Geometry check sheet. Reference: the model listing, model coordinates, mm. Round coordinates to 2 decimals unless told otherwise and drop trailing zeros. Order: outer loops, then holes, each group sorted by start corner. A loop starts at its lowest first (then second) coordinate and runs counter-clockwise, first axis right, second up. Notation, with made-up numbers: (-4, -19) - (43, -19) arc R10 cw to (43, -11) - close; hole circle Ø3 at (60.5, -18.5). An arc over 180 degrees is marked (long way). Return JSON: item names as keys, results as strings. Group by question number.
Q1. Draft check along X on faces 1 (the flat face through (5, 42, 88)), 2 (the cylindrical face through (-0.221, 63.686, 88.479)), 3 (the flat face through (0, 42, 90)). Enter one of: pulls with the +X half, pulls with the -X half, needs draft (parallel to the pull), parting line crosses it, or undercut.
Q2. Gauge pin test, flat end, axial feed: pin 1 Ø5.5 at (x, y) = (0, 22) entering from -Z. Record the tip position at first contact, or that the pin passes through.
Q3. Material ranges on line 1 along Y through (x, z) = (0, 89.2); line 2 along X through (y, z) = (22, 88.7); line 3 along Y through (x, z) = (1, 87.25), recorded low to high.
Q4. Sectioned sample at C-C, the plane z = 89.25. Record the cut outline in (x, y), then the cut area to 3 significant figures.
Q5. Sectioned sample at B-B, the plane x = 0. Record the cut outline in (y, z).
Q6. Sectioned sample at A-A, the plane y = 62. Record the cut outline in (x, z), then the cut area to 3 significant figures.
```python
from build123d import *

# Parameters (mm, degrees)
SKETCH1_W      = 10
SKETCH1_H      = 44
BAR_DEPTH      = 3
SKETCH2_R      = 1.7
M3_HOLES_DEPTH = 5


with BuildPart() as part:
    # Sketch1 → Bar (new body)
    with BuildSketch(Plane.XY.offset(87)):
        with Locations((0, 42)):
            Rectangle(SKETCH1_W, SKETCH1_H)
    extrude(amount=BAR_DEPTH)

    # Sketch2 → M3_holes (cut)
    with BuildSketch(Plane.XY.offset(86)):
        with Locations((0, 62)):
            Circle(SKETCH2_R)
        with Locations((0, 22)):
            Circle(SKETCH2_R)
    extrude(amount=M3_HOLES_DEPTH, mode=Mode.SUBTRACT)


solid = part.part
```
Reply:
{
 "1": {"face 1": "pulls with the +X half", "face 2": "undercut", "face 3": "needs draft"},
 "2": {"pin 1": "z = 87"},
 "3": {"line 1": "20 to 20.3, 23.7 to 60.3, 63.7 to 64", "line 2": "-5 to -1.7, 1.7 to 5", "line 3": "20 to 20.63, 23.37 to 60.63, 63.37 to 64"},
 "4": {"outline": "(-5, 20) - (5, 20) - (5, 64) - (-5, 64) - close; hole circle Ø3.4 at (0, 22); hole circle Ø3.4 at (0, 62)", "area": "422 mm^2"},
 "5": {"outline": "(20, 87) - (20.3, 87) - (20.3, 90) - (20, 90) - close; (23.7, 87) - (60.3, 87) - (60.3, 90) - (23.7, 90) - close; (63.7, 87) - (64, 87) - (64, 90) - (63.7, 90) - close"},
 "6": {"outline": "(-5, 87) - (-1.7, 87) - (-1.7, 90) - (-5, 90) - close; (1.7, 87) - (5, 87) - (5, 90) - (1.7, 90) - close", "area": "19.8 mm^2"}
}
